Design review of the part built by this model. Coordinates are the model's own, in mm. A direction names the side the tool comes from. Round coordinates to 2 decimals unless told otherwise and drop trailing zeros. Loops run counter-clockwise (first coordinate to the right, second up) from the corner with the lowest first, then second, coordinate; pieces in that order, holes last. Notation, with made-up numbers: (-17, 62.5) - (3, 62.5) arc R29 ccw to (3, 82.5) - close; hole circle Ø10 at (47.25, 54). An arc over 180 degrees is marked (long way). Answer as CSV lines item,"result". Start each with the question number.
(1) Consider section B-B (x = 1.8). Give the boundary of the cut face in (y, z), and give its area (3 significant figures).
(2) Wall thickness on L1, parallel to Z at x = 1.65, y = -126; L2, parallel to Y at x = 0.75, z = -4.75; L3, parallel to Z at x = 0.65, y = -127.25: over which ranges is each line inside the solid? List them lowest first.
(3) Mouldability with a two-part tool opening along Y and no side actions: class faces 1 (the cylindrical face through (1, -126.7, 3.5)), 2 (the flat face through (1, -131.8, -2)), 3 (the flat face through (0, -130.5, 0.1)) as released by +Y, released by -Y, zero draft, split by the parting line, or undercut.
(4) Consider section C-C (y = -127.25). Give the boundary of the cut face in (x, z).
(5) For P1, Ø1, axis at x = 0.5, y = -128, coming from the -Z side; P2, Ø5, axis at y = -127, z = -5, coming from the +X side (1 decimal); P3, Ø1, axis at x = 0.5, z = -5, coming from the +Y side, all flat-tipped, find the tip position at first contact; note any pin that passes through.
(6) For faces 4 (the flat face through (2, -130.5, 0.1)), 5 (the flat face through (1, -127, 2)), 6 (the flat face through (1, -133, -7)), list the 3-axis set-ups (+Z, -Z, +X, -X, +Y, -Y) from which the entire face can be reached by the end or side of a thin tool; tool diameter is ignored.
(7) Consider section A-A (z = 3.5). Give the boundary of the cut face in (x, y), and give its area (3 significant figures).
(8) Consider section D-D (z = -6). Give the boundary of the cut face in (x, y), and give its area (3 significant figures).
from build123d import *

# Parameters (mm, degrees)
EXTRUDE041_DEPTH = 2
SKETCH113_R      = 0.75
HOLE025_DEPTH    = 2
HOLE025_TIPS_R   = 0.75


with BuildPart() as part:
    # Sketch090 → Extrude041 (new body)
    with BuildSketch(Plane.YZ):
        Polygon((-128.000002, 5), (-130.000002, 5), (-130.300002, 5), (-133.300002, 5), (-133.300002, 3), (-131.800002, 3), (-131.800002, -7), (-133.300002, -7), (-133.300002, -9), (-130.300002, -9), (-130.300002, 2), (-130.000002, 2), (-128.000002, 2), (-127.700002, 2), (-124.200002, 2), (-124.200002, 5), (-127.700002, 5), align=None)
    extrude(amount=EXTRUDE041_DEPTH)

    # Sketch113 (on Face19 of Extrude041) → Hole025 (cut)
    with BuildSketch(Plane.YZ.offset(2)):
        with Locations((-125.949997, 3.5)):
            Circle(SKETCH113_R)
    extrude(amount=-HOLE025_DEPTH, mode=Mode.SUBTRACT)

    # Hole025 tips → Hole025 tip 1 section 0
    with BuildSketch(Plane.YZ, mode=Mode.PRIVATE) as hole025_tip_1_s0:
        with Locations((-125.949997, 3.5)):
            Circle(HOLE025_TIPS_R)
    loft([hole025_tip_1_s0.sketch, Vertex(-0.450645, -125.949997, 3.5)], mode=Mode.SUBTRACT)


solid = part.part
Determined:
1,outline,"(-133.3, -9) - (-130.3, -9) - (-130.3, 2) - (-124.2, 2) - (-124.2, 5) - (-133.3, 5) - (-133.3, 3) - (-131.8, 3) - (-131.8, -7) - (-133.3, -7) - close; hole circle Ø1.5 at (-125.95, 3.5)"
1,area,"43.5 mm^2"
2,L1,"z = 2 to 2.75, 4.25 to 5"
2,L2,"y = -131.8 to -130.3"
2,L3,"z = 2 to 5"
3,face 1,"undercut"
3,face 2,"released by -Y"
3,face 3,"zero draft"
4,outline,"(0, 2) - (2, 2) - (2, 5) - (0, 5) - close"
5,P1,"stops at z = 2"
5,P2,"passes through"
5,P3,"stops at y = -130.3"
6,face 4,"+Z, -Z, +X, +Y, -Y"
6,face 5,"-Z, +X, -X, +Y"
6,face 6,"+X, -X, -Y"
7,outline,"(0, -133.3) - (2, -133.3) - (2, -126.7) - (0, -126.7) - close; (0, -125.2) - (2, -125.2) - (2, -124.2) - (0, -124.2) - close"
7,area,"15.2 mm^2"
8,outline,"(0, -131.8) - (2, -131.8) - (2, -130.3) - (0, -130.3) - close"
8,area,"3.00 mm^2"
